Source: three-view drawing plus pictorial views. Frame: mm from the lowest corner of the part. A direction names the side the tool comes from. Give positions to 0.01 mm unless a question says otherwise; leave off trailing zeros. Order: outer loops, then holes, each group sorted by start corner. A loop starts at its lowest first (then second) coordinate and runs counter-clockwise, first axis right, second up. Notation, with made-up numbers: (35.5, -30.5) -> (41.5, -30.5) arc R24 ccw to (41.5, 8.5) -> close; hole circle Ø8 at (43, -39.5). An arc over 180 degrees is marked (long way). Answer in a Markdown table with one row per item.
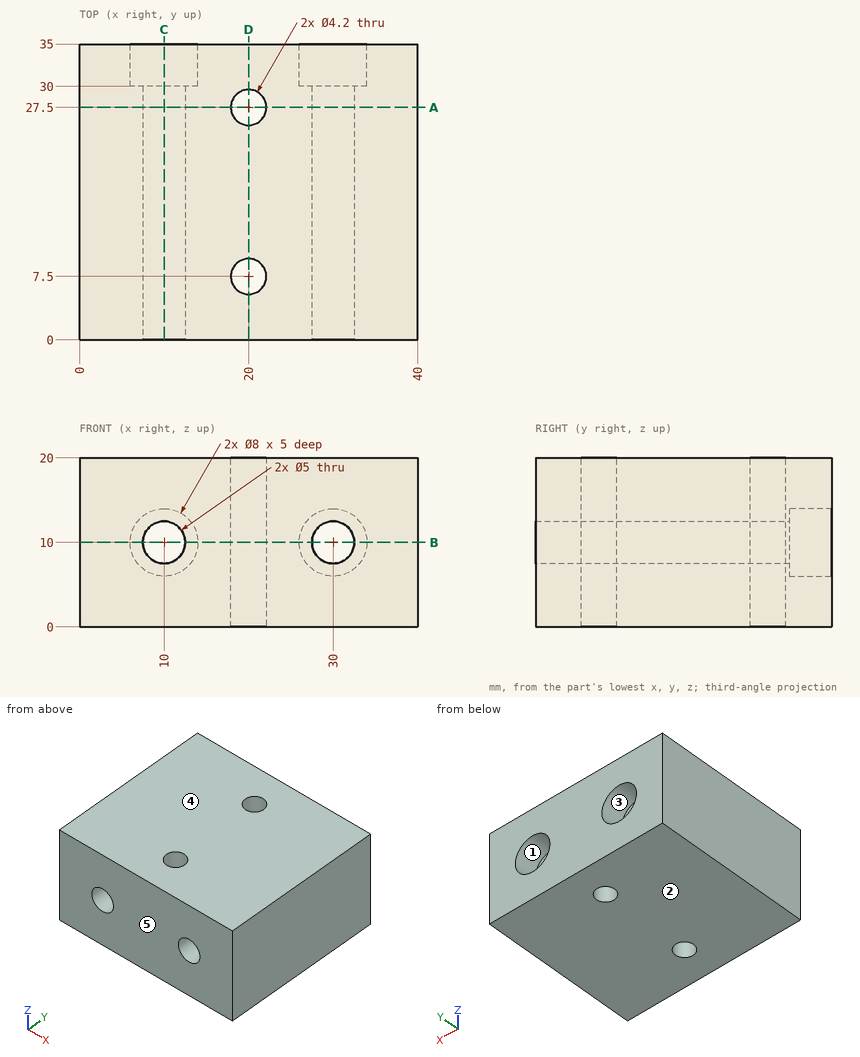
(1) Ray query, probe 1 along Y at (x, z) = (20, 6.75); probe 2 along X at (y, z) = (32.7, 10); probe 3 along X at (y, z) = (19.25, 10). Return the intervals inside material, ascending.
A:
| item | result |
|---|---|
| probe 1 | y = 0 to 5.4, 9.6 to 25.4, 29.6 to 35 |
| probe 2 | x = 0 to 6, 14 to 26, 34 to 40 |
| probe 3 | x = 0 to 7.5, 12.5 to 27.5, 32.5 to 40 |
(2) Access query for the marked faces 1 and 2. Directions: +Z, -Z, +X, -X, +Y, -Y. A direction counts if a zero-diameter tool reaches every point of the face in a straight line with its end or side. Return the directions, or none.
A:
| item | result |
|---|---|
| face 1 | +Y |
| face 2 | -Z, +X, -X, +Y, -Y |
(3) Section query D-D (x = 20). Return the cut outline in (y, z), plus the area to 3 significant figures.
A:
| item | result |
|---|---|
| outline | (0, 0) -> (5.4, 0) -> (5.4, 20) -> (0, 20) -> close; (9.6, 0) -> (25.4, 0) -> (25.4, 20) -> (9.6, 20) -> close; (29.6, 0) -> (35, 0) -> (35, 20) -> (29.6, 20) -> close |
| area | 532 mm^2 |
(4) Section query A-A (y = 27.5). Return the cut outline in (x, z).
A:
| item | result |
|---|---|
| outline | (0, 0) -> (17.9, 0) -> (17.9, 20) -> (0, 20) -> close; (22.1, 0) -> (40, 0) -> (40, 20) -> (22.1, 20) -> close; hole circle Ø5 at (10, 10); hole circle Ø5 at (30, 10) |
(5) Pull-direction query (Z, two-part tool) for the marked faces 3, 4 and 5; classes: +Z half, -Z half, draft (parallel to the pull), parting line (faces both ways), or undercut.
A:
| item | result |
|---|---|
| face 3 | undercut |
| face 4 | +Z half |
| face 5 | draft |
(6) First-contact query: pin 1 Ø2.5 at (x, z) = (31.5, 8.5) entering from +Y; pin 2 Ø4 at (x, z) = (30, 10) entering from -Y. Flat tips, straight axial feed; report the tip coordinate or a pass-through.
A:
| item | result |
|---|---|
| pin 1 | stops at y = 30 |
| pin 2 | passes through |
(7) Section query C-C (x = 10). Return the cut outline in (y, z), plus the area to 3 significant figures.
A:
| item | result |
|---|---|
| outline | (0, 0) -> (35, 0) -> (35, 6) -> (30, 6) -> (30, 7.5) -> (0, 7.5) -> close; (0, 12.5) -> (30, 12.5) -> (30, 14) -> (35, 14) -> (35, 20) -> (0, 20) -> close |
| area | 510 mm^2 |
(8) Section query B-B (z = 10). Return the cut outline in (x, y), plus the area to 3 significant figures.
A:
| item | result |
|---|---|
| outline | (0, 0) -> (7.5, 0) -> (7.5, 30) -> (6, 30) -> (6, 35) -> (0, 35) -> close; (12.5, 0) -> (27.5, 0) -> (27.5, 30) -> (26, 30) -> (26, 35) -> (14, 35) -> (14, 30) -> (12.5, 30) -> close; (32.5, 0) -> (40, 0) -> (40, 35) -> (34, 35) -> (34, 30) -> (32.5, 30) -> close; hole circle Ø4.2 at (20, 7.5); hole circle Ø4.2 at (20, 27.5) |
| area | 992 mm^2 |
